```python
from build123d import *

# Parameters (mm, degrees)
ESQUISSE1_R             = 1
BOSS_EXTRU_1_DEPTH      = 3.75
BOSS_EXTRU_1_2_DEPTH    = 3.75
BOSS_EXTRU_2_DEPTH      = 5
BOSS_EXTRU_3_DEPTH      = 2.5
BOSS_EXTRU_3_DEPTH_BACK = 2.5
BOSS_EXTRU_4_START      = -5
BOSS_EXTRU_4_DEPTH      = 5
ENL_V_MAT_EXTRU_1_DEPTH = 10


with BuildPart() as part:
    # Esquisse1 → Boss.-Extru.1 (new body)
    with BuildSketch(Plane.XY):
        with Locations((-2, 5)):
            Circle(ESQUISSE1_R)
    extrude(amount=BOSS_EXTRU_1_DEPTH)



with BuildPart() as body_2:
    # Esquisse1 → Boss.-Extru.1 2 (new body)
    with BuildSketch(Plane.XY):
        with Locations((2, -5)):
            Circle(ESQUISSE1_R)
    extrude(amount=BOSS_EXTRU_1_2_DEPTH)


with BuildPart() as part_1:
    add(part.part)

    add(body_2.part)  # Boss.-Extru.2 merges body 2
    # Esquisse2 → Boss.-Extru.2 (add)
    with BuildSketch(Plane.XY):
        with BuildLine():
            Line((-5.5, -10), (5.5, -10))
            ThreePointArc((5.5, -10), (6.914213562, -9.414213562), (7.5, -8))
            Line((7.5, -8), (7.5, 8))
            ThreePointArc((7.5, 8), (6.914213562, 9.414213562), (5.5, 10))
            Line((5.5, 10), (-5.5, 10))
            ThreePointArc((-5.5, 10), (-6.914213562, 9.414213562), (-7.5, 8))
            Line((-7.5, 8), (-7.5, -8))
            ThreePointArc((-7.5, -8), (-6.914213562, -9.414213562), (-5.5, -10))
        make_face()
    extrude(amount=-BOSS_EXTRU_2_DEPTH)

    # Esquisse3 → Boss.-Extru.3 (add, two sides: drawn at the far end of the back side and taken through both)
    with BuildSketch(Plane(origin=(0, 0, 0), x_dir=(1, 0, 0), z_dir=(0, 1, 0)).offset(-BOSS_EXTRU_3_DEPTH_BACK)):
        Polygon((-15.908235074, 13.872743974), (-15.908235074, 15.554043285), (-3.755300915, 15.554043285), (2, 5), (-2, 5), (-6.838459549, 13.872743974), align=None)
    extrude(amount=BOSS_EXTRU_3_DEPTH + BOSS_EXTRU_3_DEPTH_BACK)

    # Esquisse4 → Boss.-Extru.4 (add)
    with BuildSketch(Plane.XZ.offset(2.5).offset(BOSS_EXTRU_4_START)):
        Polygon((-9.831767995, -15.554043285), (-24.998481753, -28.725072904), (-74.998481753, -28.725072904), (-74.998481753, -22.039407789), (-24.998481753, -22.039407789), (-15.908235074, -13.872743974), align=None)
    extrude(amount=BOSS_EXTRU_4_DEPTH)

    # Esquisse6 → Enlèv. mat.-Extru.1 (cut)
    with BuildSketch(Plane(origin=(0, 0, -28.725072904), x_dir=(-1, 0, 0), z_dir=(0, 0, -1))):
        Polygon((39.752900497, -2.5), (39.752900497, 2.5), (50.637754923, 9.880645694), (75.638904933, 6.190322847), (75.638904933, -4.915953291), (39.752900497, -8.60093005), align=None)
    extrude(amount=-ENL_V_MAT_EXTRU_1_DEPTH, mode=Mode.SUBTRACT)


solid = part_1.part
```
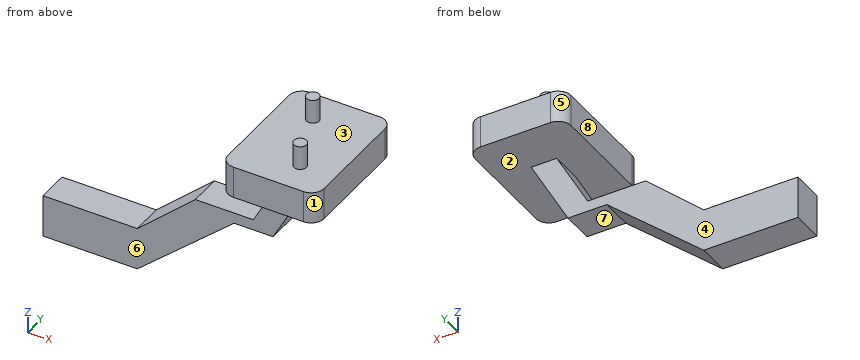
Model file for the job. Use its own axes, mm. Face numbers are marked on the shaded views. A direction names the side the tool comes from. Give positions to 0.01 mm unless a question says otherwise; leave off trailing zeros. Loops run counter-clockwise (first coordinate to the right, second up) from the corner with the lowest first, then second, coordinate; pieces in that order, holes last. Notation, with made-up numbers: M 17.5,1.5 L 56.5,1.5 A33 cw 56.5,29.5 Z; hole C 11,29.25 d10. An arc over 180 degrees is marked long. Use one line per item in the form item = value.
Item 1: Slice it at B-B on y = -5. List the corners of the cut face in (x, z), and give its area (3 significant figures).
Filled in:
outline = M -7.5,-5 L 7.5,-5 L 7.5,0 L 3,0 L 3,3.75 L 1,3.75 L 1,0 L -7.5,0 Z
area = 82.5 mm^2
Item 2: Two-plate mould, pull along Z, no slides. Class the marked faces 1, 2 and 3: released by +Z, released by -Z, zero draft, split by the parting line, or undercut.
Filled in:
face_1 = zero draft
face_2 = undercut
face_3 = released by +Z
Item 3: Slice it at D-D on y = -1.25. List the corners of the cut face in (x, z), and give its area (3 significant figures).
Filled in:
outline = M -39.75,-28.73 L -25,-28.73 L -9.83,-15.55 L -3.76,-15.55 L 2,-5 L 7.5,-5 L 7.5,0 L -7.5,0 L -7.5,-5 L -2,-5 L -6.84,-13.87 L -15.91,-13.87 L -25,-22.04 L -39.75,-22.04 Z
area = 308 mm^2
Item 4: Flat gauge pins, fed straight in: pin 1 Ø12 at (x, y) = (-9.5, -6.5) entering from +Z; pin 2 Ø5.5 at (x, y) = (-8, -0.5) entering from -Z; pin 3 Ø12 at (x, y) = (-3.5, -0.5) entering from -Z; pin 4 Ø1.5 at (x, y) = (-8.5, -5.5) entering from +Z. Where does each tip first touch, or does it go through?
Filled in:
pin_1 = 0
pin_2 = -16.35
pin_3 = -15.55
pin_4 = through
Item 5: Drill centre lines: L1, parallel to Z at x = 4.5, y = 0.5; L2, parallel to Z at x = -30, y = -2; L3, parallel to Y at x = -5.5, z = -12. Where is each one in solid material? Low to high.
Filled in:
L1 = -5 to 0
L2 = -28.73 to -22.04
L3 = -2.5 to 2.5
Item 6: Slice it at C-C on x = 4. List the corners of the cut face in (y, z), and give its area (3 significant figures).
Filled in:
outline = M -10,-5 L 10,-5 L 10,0 L -10,0 Z
area = 100 mm^2
Item 7: Slice it at A-A on x = -4.5. List the corners of the cut face in (y, z).
Filled in:
outline = M -10,-5 L 10,-5 L 10,0 L -10,0 Z; M -2.5,-15.55 L 2.5,-15.55 L 2.5,-9.58 L -2.5,-9.58 Z
Item 8: Which spindle directions (+Z, -Z, +X, -X, +Y, -Y) get a long thin tool onto all of the face, cutting with end or side? Do the marked faces 4, 5, 6, 7 and 8. Say none if no direction does.
Filled in:
face_4 = -Z, +X, -X, +Y
face_5 = +Z, -Z, -X, +Y
face_6 = -Z, +X, -X, -Y
face_7 = -Z, +X, +Y, -Y
face_8 = +Z, -X, +Y, -Y
